Part model, mm, in its own coordinate system. A direction names the side the tool comes from. Give positions to 0.01 mm unless a question says otherwise; leave off trailing zeros. Order: outer loops, then holes, each group sorted by start corner. A loop starts at its lowest first (then second) coordinate and runs counter-clockwise, first axis right, second up. Notation, with made-up numbers: M -36.5,-24.75 L -21.5,-24.75 A35 ccw -21.5,9.25 Z; hole C 7,-27 d7. An arc over 180 degrees is marked long. Answer as a JSON object with one key per item and string values.
from build123d import *

# Parameters (mm, degrees)
F0_R        = 10.16
F1_DEPTH    = 1.5875
F2_R        = 4
F3_DEPTH    = 8
F5_DEPTH    = 8
F6_R        = 5.715
F7_DEPTH    = 0.5
F9_DEPTH    = 1.5875
F10_SIZE2   = 1.5748
F10_SIZE    = 0.79375
F10_2_SIZE2 = 1.5748
F10_2_SIZE  = 0.79375
F10_3_SIZE2 = 1.5748
F10_3_SIZE  = 0.79375
F12_DEPTH   = 2.0885
F13_R       = 1


with BuildPart() as f1:
    # F0 (on Top) → F1 (new body)
    with BuildSketch(Plane.XY):
        Circle(F0_R)
    extrude(amount=F1_DEPTH)

    # F2 (on face) → F3 (join)
    with BuildSketch(Plane.XY.offset(1.5875)):
        Circle(F2_R)
        Polygon((0, 3.6661742094), (3.175, 1.8330871047), (3.175, -1.8330871047), (0, -3.6661742094), (-3.175, -1.8330871047), (-3.175, 1.8330871047), align=None, mode=Mode.SUBTRACT)
        Polygon((-0.5826233556, 0), (-3.175, 1.8330871047), (-3.175, -1.8330871047), align=None)
        Polygon((0.2913116778, 0.5045666267), (3.175, 1.8330871047), (0, 3.6661742094), align=None)
        Polygon((0, -3.6661742094), (3.175, -1.8330871047), (0.2913116778, -0.5045666267), align=None)
    extrude(amount=F3_DEPTH)

    # F4 (on face) → F5 (cut, through all)
    with BuildSketch(Plane.XY.offset(9.5875)):
        with BuildLine():
            Line((-3.175, 1.8330871047), (0, 3.6661742094))
            Line((0, 3.6661742094), (0.1901242338, 3.9954790421))
            ThreePointArc((0.1901242338, 3.9954790421), (-2, 3.4641016151), (-3.5552484676, 1.8330871047))
            Line((-3.5552484676, 1.8330871047), (-3.175, 1.8330871047))
        make_face()
        with BuildLine():
            Line((3.3651242338, 2.1623919374), (3.175, 1.8330871047))
            Line((3.175, 1.8330871047), (3.175, -1.8330871047))
            Line((3.175, -1.8330871047), (3.3651242338, -2.1623919374))
            ThreePointArc((3.3651242338, -2.1623919374), (3.838000582, -1.1268325219), (4, 0))
            ThreePointArc((4, 0), (3.838000582, 1.1268325219), (3.3651242338, 2.1623919374))
        make_face()
        with BuildLine():
            Line((0, -3.6661742094), (-3.175, -1.8330871047))
            Line((-3.175, -1.8330871047), (-3.5552484676, -1.8330871047))
            ThreePointArc((-3.5552484676, -1.8330871047), (-2, -3.4641016151), (0.1901242338, -3.9954790421))
            Line((0.1901242338, -3.9954790421), (0, -3.6661742094))
        make_face()
    extrude(amount=-F5_DEPTH, mode=Mode.SUBTRACT)

    # F6 (on face) → F7 (join)
    with BuildSketch(Plane.XY.offset(1.5875)):
        Circle(F6_R)
    extrude(amount=F7_DEPTH)

    # F8 (on face) → F9 (join)
    with BuildSketch(Plane.XY.offset(9.5875)):
        Polygon((-3.175, -1.8330871047), (-0.5826233556, 0), (-3.175, 1.8330871047), (-3.5552484676, 1.8330871047), (-3.5552484676, -1.8330871047), align=None)
        with BuildLine():
            ThreePointArc((-3.5552484676, 1.8330871047), (-4, 0), (-3.5552484676, -1.8330871047))
            Line((-3.5552484676, -1.8330871047), (-3.5552484676, 1.8330871047))
        make_face()
        with BuildLine():
            Line((-4.7377411988, -1.8330871047), (-3.5552484676, -1.8330871047))
            ThreePointArc((-3.5552484676, -1.8330871047), (-4, 0), (-3.5552484676, 1.8330871047))
            Line((-3.5552484676, 1.8330871047), (-4.7377411988, 1.8330871047))
            ThreePointArc((-4.7377411988, 1.8330871047), (-5.08, 0), (-4.7377411988, -1.8330871047))
        make_face()
        Polygon((0.1901242338, 3.9954790421), (0, 3.6661742094), (0.2913116778, 0.5045666267), (3.175, 1.8330871047), (3.3651242338, 2.1623919374), align=None)
        with BuildLine():
            ThreePointArc((3.3651242338, 2.1623919374), (2, 3.4641016151), (0.1901242338, 3.9954790421))
            Line((0.1901242338, 3.9954790421), (3.3651242338, 2.1623919374))
        make_face()
        with BuildLine():
            Line((0.7813705994, 5.019547787), (0.1901242338, 3.9954790421))
            ThreePointArc((0.1901242338, 3.9954790421), (2, 3.4641016151), (3.3651242338, 2.1623919374))
            Line((3.3651242338, 2.1623919374), (3.9563705994, 3.1864606824))
            ThreePointArc((3.9563705994, 3.1864606824), (2.54, 4.3994090512), (0.7813705994, 5.019547787))
        make_face()
        Polygon((3.175, -1.8330871047), (0.2913116778, -0.5045666267), (0, -3.6661742094), (0.1901242338, -3.9954790421), (3.3651242338, -2.1623919374), align=None)
        with BuildLine():
            ThreePointArc((0.1901242338, -3.9954790421), (2, -3.4641016151), (3.3651242338, -2.1623919374))
            Line((3.3651242338, -2.1623919374), (0.1901242338, -3.9954790421))
        make_face()
        with BuildLine():
            Line((3.9563705994, -3.1864606824), (3.3651242338, -2.1623919374))
            ThreePointArc((3.3651242338, -2.1623919374), (2, -3.4641016151), (0.1901242338, -3.9954790421))
            Line((0.1901242338, -3.9954790421), (0.7813705994, -5.019547787))
            ThreePointArc((0.7813705994, -5.019547787), (2.54, -4.3994090512), (3.9563705994, -3.1864606824))
        make_face()
    extrude(amount=F9_DEPTH)

    # F10
    f10_edges = [f1.edges().sort_by_distance(p)[0] for p in [
        (2.54, -4.399409, 11.175),
    ]]
    f10_side = f1.faces().sort_by_distance((1.667082, -2.88747, 11.175))[0]
    chamfer(f10_edges, length=F10_SIZE, length2=F10_SIZE2, reference=f10_side)

    # F10#2
    f10_2_edges = [f1.edges().sort_by_distance(p)[0] for p in [
        (2.54, 4.399409, 11.175),
    ]]
    f10_2_side = f1.faces().sort_by_distance((1.667082, 2.88747, 11.175))[0]
    chamfer(f10_2_edges, length=F10_2_SIZE, length2=F10_2_SIZE2, reference=f10_2_side)

    # F10#3
    f10_3_edges = [f1.edges().sort_by_distance(p)[0] for p in [
        (-5.08, 0, 11.175),
    ]]
    f10_3_side = f1.faces().sort_by_distance((-3.334164, 0, 11.175))[0]
    chamfer(f10_3_edges, length=F10_3_SIZE, length2=F10_3_SIZE2, reference=f10_3_side)

    # F11 (on face) → F12 (cut, through all)
    with BuildSketch(Plane.XY.offset(2.0875)):
        with BuildLine():
            ThreePointArc((4.4630241186, -2.4264821691), (4.9233404576, -1.2518461322), (5.08, 0))
            ThreePointArc((5.08, 0), (4.9233404576, 1.2518461322), (4.4630241186, 2.4264821691))
            Line((4.4630241186, 2.4264821691), (3.175, 1.8330871047))
            Line((3.175, 1.8330871047), (0.2913116778, 0.5045666267))
            Line((0.2913116778, 0.5045666267), (0, 3.6661742094))
            Line((0, 3.6661742094), (-0.1301168591, 5.0783333489))
            ThreePointArc((-0.1301168591, 5.0783333489), (-2.54, 4.3994090512), (-4.3329072595, 2.6518511799))
            Line((-4.3329072595, 2.6518511799), (-3.175, 1.8330871047))
            Line((-3.175, 1.8330871047), (-0.5826233556, 0))
            Line((-0.5826233556, 0), (-3.175, -1.8330871047))
            Line((-3.175, -1.8330871047), (-4.3329072595, -2.6518511799))
            ThreePointArc((-4.3329072595, -2.6518511799), (-2.54, -4.3994090512), (-0.1301168591, -5.0783333489))
            Line((-0.1301168591, -5.0783333489), (0, -3.6661742094))
            Line((0, -3.6661742094), (0.2913116778, -0.5045666267))
            Line((0.2913116778, -0.5045666267), (3.175, -1.8330871047))
            Line((3.175, -1.8330871047), (4.4630241186, -2.4264821691))
        make_face()
    extrude(amount=-F12_DEPTH, mode=Mode.SUBTRACT)

    # F13
    f13_edges = [f1.edges().sort_by_distance(p)[0] for p in [
        (-10.16, 0, 0),
    ]]
    fillet(f13_edges, radius=F13_R)


solid = f1.part
1. Which spindle directions (+Z, -Z, +X, -X, +Y, -Y) get a long thin tool onto all of the face, cutting with end or side? Do faces 4 (the cylindrical face through (2.023, 3.451, 5.785)), 5 (the cylindrical face through (5.45, 1.72, 1.83)), 6 (the flat face through (2, -4, 9.588)), 7 (the flat face through (-4, 2, 2.088)), 8 (the cylindrical face through (-2.509, 4.417, 1.058)). Say none if no direction does.
Worked answers:
{"face 4": "+X, +Y", "face 5": "+Z", "face 6": "+X, -Y", "face 7": "none", "face 8": "+Z, -Z"}
2. Probe line 1 along Y through (x, z) = (-2.25, 2); line 2 along Y through (x, z) = (1, 8.5); line 3 along Y through (x, z) = (2.75, 3.75). List the from-to ranges inside material, lowest first.
Worked answers:
{"line 1": "y = -5.25 to -4.55, -1.18 to 1.18, 4.55 to 5.25", "line 2": "y = -3.87 to -0.83, 0.83 to 3.87", "line 3": "y = -2.9 to -1.64, 1.64 to 2.9"}
3. Pin check, flat tips, straight feed: P1, Ø5, axis at y = -6.5, z = 1.5, coming from the +X side; P2, Ø1.3, axis at x = -4, z = 4.5, coming from the +Y side; P3, Ø1.5, axis at x = -2, z = 8, coming from the +Y side. Stop position of each tip, or through.
Worked answers:
{"P1": "stops at x = 9.34", "P2": "stops at y = 1.83", "P3": "stops at y = 1.53"}
4. Cut at A-A on z = 4.5. Give the cut face in (x, y) (3 decimals).
Worked answers:
{"outline": "M -3.555,-1.833 L -3.175,-1.833 L -0.583,0 L -3.175,1.833 L -3.555,1.833 A4 ccw Z; M 0,-3.666 L 0.19,-3.995 A4 ccw 3.365,-2.162 L 3.175,-1.833 L 0.291,-0.505 Z; M 0,3.666 L 0.291,0.505 L 3.175,1.833 L 3.365,2.162 A4 ccw 0.19,3.995 Z"}
5. Two-plate mould, pull along Z, no slides. Class faces 1 (the cylindrical face through (1.977, -3.477, 5.785)), 2 (the cylindrical face through (-2.57, -4.38, 1.06)), 3 (the flat face through (-2, 0, 0)): +Z half, -Z half, draft (parallel to the pull), parting line (faces both ways), or undercut.
Worked answers:
{"face 1": "undercut", "face 2": "draft", "face 3": "-Z half"}
6. Cut at B-B on y = -1.5. State how many separate pieces and enclosed holes the cut face has, plus the area to 3 significant figures.
Worked answers:
{"separate pieces": "3", "enclosed holes": "0", "area": "56.7 mm^2"}
